Source: CAD feature listing. Evaluate the final solid. Frame: model axes, mm. A direction names the side the tool comes from. Give positions to 0.01 mm unless a question says otherwise; leave off trailing zeros.
1) Access query for faces 4 (the face through (183.677, -318.255, 291.831)), 5 (the face through (12.131, -327.544, 251.152)), 6 (the face through (66.28, 427.61, 134.66)). Directions: +Z, -Z, +X, -X, +Y, -Y. A direction counts if a zero-diameter tool reaches every point of the face in a straight line with its end or side. Return the directions, or none.
2) Draft query along X for faces 1 (the face through (202.82, -55.24, -420.75)), 2 (the face through (26.399, -100.489, -452.527)), 3 (the face through (77.837, -97.391, -438.58)). Return one class per face: released by +X, released by -X, zero draft, split by the parting line, or undercut.
3) Material intervals for line 1 (X direction, y = 322, z = 332.5); line 2 (Z direction, x = 12, y = 0); line 3 (Z direction, x = 93.5, y = 0) (3 decimals), sorted ascending.
4) First-contact query: P1, Ø4, axis at x = 33.5, y = -47, coming from the -Z side; P2, Ø12, axis at x = 39.5, z = 73.5, coming from the +Y side; P3, Ø8, axis at x = 23.5, y = -282.5, coming from the -Z side. Flat tips, straight axial feed; report the tip coordinate or a pass-through.
Autodesk Inventor part; units mm, degrees
ref_plane "YZ Plane" through (0, 0, 0) normal (1, 0, 0) x (0, 1, 0)
ref_plane "XZ Plane" through (0, 0, 0) normal (0, 1, 0) x (-1, 0, 0)
ref_plane "XY Plane" through (0, 0, 0) normal (0, 0, 1) x (1, 0, 0)
sketch "Sketch1" plane through (0, 0, 0) normal (0, 0, 1) x (1, 0, 0)
  line L0 (0, 412.75) -> (0, 463.55)
  line L1 (0, 463.55) -> (52.07, 463.55)
  line L2 (52.07, 463.55) -> (54.7572, 448.31)
  line L3 (54.7572, 448.31) -> (77.4902, 448.31)
  line L4 (77.4902, 448.31) -> (83.0371, 463.55)
  line L5 (83.0371, 463.55) -> (157.1625, 463.55)
  line L6 (169.8625, 431.8) -> (197.1093, 431.8)
  line L7 (197.1093, 431.8) -> (203.2, 423.8625)
  line L8 (203.2, 422.275) -> (157.1625, 422.275)
  line L9 (25.4, 415.925) -> (25.4, 412.75)
  line L10 (25.4, 412.75) -> (0, 412.75)
  arc A0 (31.75, 422.275) -> (25.4, 415.925) centre (31.75, 415.925) ccw
  line L11 (-40.64, 0) -> (243.84, 0)
  line L12 (203.2, 422.275) -> (203.2, 423.8625)
  line L13 (31.75, 422.275) -> (157.1625, 422.275)
  line L14 (157.1625, 463.55) -> (157.1625, 444.5)
  arc A1 (157.1625, 444.5) -> (169.8625, 431.8) centre (169.8625, 444.5) ccw
  point P0 (0, 0)
  dimension "d0" = 463.55
  dimension "d3" = 431.8
  dimension "d5" = 7.9375
  dimension "d10" = 6.35
  dimension "d12" = 412.75
  dimension "d13" = 52.07
  dimension "d17" = 9.525
  dimension "d35" = 25.4
  dimension "d38" = 10
  dimension "d39" = 20
  dimension "d40" = 22.733
  dimension "d41" = 15.24
  dimension "d44" = 203.2
  dimension "d45" = 37.5
  dimension "d55" = 422.275
  dimension "d58" = 12.7
  dimension "d59" = 157.1625
revolve "Revolution1" add sketch "Sketch1" angle 360 about axis through (-10, 0, 0) along (1, 0, 0)
chamfer "Chamfer2" distance 0.7937 angle 45 2 edges at (25.4, -415.925, 0) (25.4, -412.75, 0)
properties part number "A1-19027-400-04 34in Type B Victaulic ring" material "Steel, Mild"
From the geometry:
1. face 4: +X
1. face 5: +X, -X
1. face 6: none
2. face 1: released by +X
2. face 2: zero draft
2. face 3: undercut
3. line 1: x = 0 to 52.19, 82.79 to 157.16
3. line 2: z = -463.55 to -412.75, 412.75 to 463.55
3. line 3: z = -463.55 to -422.275, 422.275 to 463.55
4. P1: stops at z = -461.36
4. P2: stops at y = 458.61
4. P3: stops at z = -370.56
